Could you check a few things on this model? Use its own coordinates, in mm. A direction names the side the tool comes from. Give positions to 0.01 mm unless a question says otherwise; leave off trailing zeros. Write each loop counter-clockwise with the first axis right and the second up, starting at its lowest first coordinate (ties: lowest second). Pieces come first, ordered by that corner, then holes. Notation, with made-up numbers: (71.25, 7.25) - (85.25, 7.25) arc R32 ccw to (85.25, 33.25) - close; hole circle Ø8 at (-12, -14.75). An arc over 180 degrees is marked (long way). Answer in a Markdown table with one row per item.
from build123d import *
from OCP.BRepFilletAPI import BRepFilletAPI_MakeChamfer

# Parameters (mm, degrees)
ESTRUSIONE_ESTRUSIONE1_DEPTH                         = 66
RACCORDO1_R                                          = 10
SMUSSO1_SIZE                                         = 2
SMUSSO1_SIZE2                                        = 2.155800013
SMUSSO1_SIZE2_2                                      = 1.873732722
SMUSSO2_SIZE                                         = 5
FORO_LAMATO_PER_VITE_M4_A_TESTA_CILINDRI_D           = 4.5
FORO_LAMATO_PER_VITE_M4_A_TESTA_CILINDRI_DEPTH       = 30
FORO_LAMATO_PER_VITE_M4_A_TESTA_CILINDRI_CBORE_D     = 10
FORO_LAMATO_PER_VITE_M4_A_TESTA_CILINDRI_CBORE_DEPTH = 3
FORO_LAMATO_PER_VITE_M4_A_TESTA_CILINDRI_TIP         = 1.351936393
FORO_LAMATO_PER_VITE_M4_A_TESTA_CILI_2_D             = 4.5
FORO_LAMATO_PER_VITE_M4_A_TESTA_CILI_2_DEPTH         = 30
FORO_LAMATO_PER_VITE_M4_A_TESTA_CILI_2_CBORE_D       = 10
FORO_LAMATO_PER_VITE_M4_A_TESTA_CILI_2_CBORE_DEPTH   = 10
FORO_LAMATO_PER_VITE_M4_A_TESTA_CILI_2_TIP           = 1.351936393
FORO_LAMATO_PER_VITE_M4_A_TESTA_CILI_3_D             = 4.5
FORO_LAMATO_PER_VITE_M4_A_TESTA_CILI_3_DEPTH         = 45
FORO_LAMATO_PER_VITE_M4_A_TESTA_CILI_3_CBORE_D       = 10
FORO_LAMATO_PER_VITE_M4_A_TESTA_CILI_3_CBORE_DEPTH   = 32
FORO_LAMATO_PER_VITE_M4_A_TESTA_CILI_3_TIP           = 1.351936393


with BuildPart() as part:
    # Schizzo1 → Estrusione-Estrusione1 (new body)
    with BuildSketch(Plane.XY):
        Polygon((25.25, 100), (32.25, 100), (39.25, 0), (-39.25, 0), (-64.110342, 0), (-64.110342, 114.69), (-25.25, 114.69), (-25.25, 100), (-25.25, 15), (25.25, 15), align=None)
    extrude(amount=ESTRUSIONE_ESTRUSIONE1_DEPTH)

    # Raccordo1
    raccordo1_edges = [part.edges().sort_by_distance(p)[0] for p in [
        (-25.25, 15, 33),
        (25.25, 15, 33),
    ]]
    fillet(raccordo1_edges, radius=RACCORDO1_R)

    # Smusso1: one chamfer whose edges measure the first distance from different faces: ONE call of the kernel's chamfer builder (chamfer() names one face for all edges)
    smusso1_edges_1 = [part.edges().sort_by_distance(p)[0] for p in [
        (35.75, 50, 0),
        (-12.430171, 0, 0),
        (-64.110342, 57.345, 0),
        (-44.680171, 114.69, 0),
        (25.25, 62.5, 0),
        (25.25, 100, 33),
        (-44.680171, 114.69, 66),
        (-64.110342, 57.345, 66),
        (-12.430171, 0, 66),
        (-25.25, 69.845, 0),
        (-25.25, 69.845, 66),
        (0, 15, 0),
        (0, 15, 66),
        (-22.321067812, 17.928932188, 0),
        (-22.321067812, 17.928932188, 66),
        (35.75, 50, 66),
        (22.321067812, 17.928932188, 0),
        (22.321067812, 17.928932188, 66),
        (25.25, 62.5, 66),
    ]]
    smusso1_edges_2 = [part.edges().sort_by_distance(p)[0] for p in [
        (32.25, 100, 33),
    ]]
    smusso1_side_2 = [part.faces().sort_by_distance(p)[0] for p in [
        (35.75, 50, 33),
    ]]
    smusso1_edges_3 = [part.edges().sort_by_distance(p)[0] for p in [
        (39.25, 0, 33),
    ]]
    smusso1_side_3 = [part.faces().sort_by_distance(p)[0] for p in [
        (-12.430171, 0, 33),
    ]]
    smusso1 = BRepFilletAPI_MakeChamfer(part.part.solid().wrapped)
    for e in smusso1_edges_1:
        smusso1.Add(SMUSSO1_SIZE, e.wrapped)
    for e in smusso1_edges_2:
        smusso1.Add(SMUSSO1_SIZE, SMUSSO1_SIZE2, e.wrapped, smusso1_side_2[0].wrapped)  # the first distance lies on this face
    for e in smusso1_edges_3:
        smusso1.Add(SMUSSO1_SIZE, SMUSSO1_SIZE2_2, e.wrapped, smusso1_side_3[0].wrapped)  # the first distance lies on this face
    add(Compound.cast(smusso1.Shape()), mode=Mode.REPLACE)

    # Smusso2
    # the kernel refuses this chamfer: 5 mm, written as the material it takes off along each edge
    with BuildSketch(Plane(origin=(14.39158506, 100, 66), x_dir=(2.02935454733688e-15, -0.9996219169112968, 0.027495876610587663), z_dir=(1, 0, 0)), Plane(origin=(14.39158506, 100, 0), x_dir=(0, 0.0274958766105877, 0.9996219169112968), z_dir=(1, 0, 0))) as smusso2_piece_1:
        Polygon((SMUSSO2_SIZE * 0.999621916911, SMUSSO2_SIZE * 0.0274958766106), (-SMUSSO2_SIZE * 0.0274958766106, SMUSSO2_SIZE * 0.999621916911), (0, 0), align=None)
    extrude(amount=28.561029867, mode=Mode.SUBTRACT)

    # Foro lamato per Vite M4 a testa cilindri
    with Locations(Plane(origin=(35.25, 0, 0), x_dir=(0, 0, 1), z_dir=(1, 0, 0))):
        with Locations((56, -85.613628), (10, -85.613628)):
            CounterBoreHole(FORO_LAMATO_PER_VITE_M4_A_TESTA_CILINDRI_D / 2, FORO_LAMATO_PER_VITE_M4_A_TESTA_CILINDRI_CBORE_D / 2, FORO_LAMATO_PER_VITE_M4_A_TESTA_CILINDRI_CBORE_DEPTH, depth=FORO_LAMATO_PER_VITE_M4_A_TESTA_CILINDRI_DEPTH)
            with Locations((0, 0, -(FORO_LAMATO_PER_VITE_M4_A_TESTA_CILINDRI_DEPTH + FORO_LAMATO_PER_VITE_M4_A_TESTA_CILINDRI_TIP / 2))):  # 118° drill point
                Cone(0, FORO_LAMATO_PER_VITE_M4_A_TESTA_CILINDRI_D / 2, FORO_LAMATO_PER_VITE_M4_A_TESTA_CILINDRI_TIP, mode=Mode.SUBTRACT)

    # Foro lamato per Vite M4 a testa cili 2
    with Locations(Plane(origin=(0, 15, 0), x_dir=(1, 0, 0), z_dir=(0, 1, 0))):
        with Locations((-10.245584981, -33), (9.754415019, -33)):
            CounterBoreHole(FORO_LAMATO_PER_VITE_M4_A_TESTA_CILI_2_D / 2, FORO_LAMATO_PER_VITE_M4_A_TESTA_CILI_2_CBORE_D / 2, FORO_LAMATO_PER_VITE_M4_A_TESTA_CILI_2_CBORE_DEPTH, depth=FORO_LAMATO_PER_VITE_M4_A_TESTA_CILI_2_DEPTH)
            with Locations((0, 0, -(FORO_LAMATO_PER_VITE_M4_A_TESTA_CILI_2_DEPTH + FORO_LAMATO_PER_VITE_M4_A_TESTA_CILI_2_TIP / 2))):  # 118° drill point
                Cone(0, FORO_LAMATO_PER_VITE_M4_A_TESTA_CILI_2_D / 2, FORO_LAMATO_PER_VITE_M4_A_TESTA_CILI_2_TIP, mode=Mode.SUBTRACT)

    # Foro lamato per Vite M4 a testa cili 3
    with Locations(Plane.ZY.offset(64.110342)):
        with Locations((10, 85.613628), (56, 85.613628)):
            CounterBoreHole(FORO_LAMATO_PER_VITE_M4_A_TESTA_CILI_3_D / 2, FORO_LAMATO_PER_VITE_M4_A_TESTA_CILI_3_CBORE_D / 2, FORO_LAMATO_PER_VITE_M4_A_TESTA_CILI_3_CBORE_DEPTH, depth=FORO_LAMATO_PER_VITE_M4_A_TESTA_CILI_3_DEPTH)
            with Locations((0, 0, -(FORO_LAMATO_PER_VITE_M4_A_TESTA_CILI_3_DEPTH + FORO_LAMATO_PER_VITE_M4_A_TESTA_CILI_3_TIP / 2))):  # 118° drill point
                Cone(0, FORO_LAMATO_PER_VITE_M4_A_TESTA_CILI_3_D / 2, FORO_LAMATO_PER_VITE_M4_A_TESTA_CILI_3_TIP, mode=Mode.SUBTRACT)


solid = part.part
1) Imagine slicing it at C-C (y = 9). List the corners of the cut face in (x, z) for me, then the cut area to 3 significant figures.
Check values:
| item | result |
|---|---|
| outline | (-64.11, 2) - (-62.11, 0) - (36.62, 0) - (38.62, 2) - (38.62, 64) - (36.62, 66) - (-62.11, 66) - (-64.11, 64) - close; hole circle Ø10 at (-10.25, 33); hole circle Ø10 at (9.75, 33) |
| area | 6,620 mm2 |
2) On a 3-axis mill with a long thin cutter (end or side, diameter ignored), from which of +Z, -Z, +X, -X, +Y, -Y can I reach the whole of each face in a straight line? I mean faces 5 (the face through (32.815, 80.656, 55.349)), 6 (the face through (29, 98, 3)), 7 (the face through (-22.786, 17.628, 1.458)). Say none if no direction works.
Check values:
| item | result |
|---|---|
| face 5 | +X |
| face 6 | -Z, +X, +Y |
| face 7 | -Z, +Y |
3) Imagine slicing it at A-A (z = 33). State how many separate pieces and enclosed holes the cut face has, then the cut area to 3 significant figures.
Check values:
| item | result |
|---|---|
| separate pieces | 3 |
| enclosed holes | 0 |
| area | 6,060 mm2 |
4) Will these pins go through, and if not, where does the flat tip stop? P1, Ø11.5, axis at x = -10.25, z = 33, coming from the +Y side; P2, Ø8, axis at y = 86, z = 54.5, coming from the +X side; P3, Ø5, axis at y = 41.5, z = 49, coming from the +X side.
Check values:
| item | result |
|---|---|
| P1 | stops at y = 15.03 |
| P2 | stops at x = 33.42 |
| P3 | stops at x = 36.52 |
5) Imagine slicing it at D-D (x = -38.5). List the corners of the cut face in (y, z) for me, then the cut area to 3 significant figures.
Check values:
| item | result |
|---|---|
| outline | (0, 2) - (2, 0) - (112.69, 0) - (114.69, 2) - (114.69, 64) - (112.69, 66) - (2, 66) - (0, 64) - close; hole circle Ø10 at (85.61, 10); hole circle Ø10 at (85.61, 56) |
| area | 7,400 mm2 |
6) If I drill on line 1 (Y direction, x = -46, z = 56); line 2 (X direction, y = 88, z = 7); line 3 (Y direction, x = 30, z = 56), over which ranges is the centre line in solid material (lowest first)?
Check values:
| item | result |
|---|---|
| line 1 | y = 0 to 80.61, 90.61 to 114.69 |
| line 2 | x = -32.11 to -25.25, 25.25 to 32.25 |
| line 3 | y = 0 to 83.36, 87.86 to 100 |
7) Imagine slicing it at B-B (z = 21.5). List the corners of the cut face in (x, y) for me, then the cut area to 3 significant figures.
Check values:
| item | result |
|---|---|
| outline | (-64.11, 0) - (37.25, 0) - (39.12, 1.87) - (32.39, 98) - (30.09, 100) - (27.25, 100) - (25.25, 98) - (25.25, 25) arc R10 cw to (15.25, 15) - (-15.25, 15) arc R10 cw to (-25.25, 25) - (-25.25, 114.69) - (-64.11, 114.69) - close |
| area | 6,300 mm2 |
8) We'd pull the mould along Y, two halves only. Please class faces 1 (the face through (-48.334, 87.115, 14.769)), 2 (the face through (25.25, 61, 33)), 3 (the face through (28.7, 87.81, 10.49)), 4 (the face through (-45, 114.69, 33)): +Y half, -Y half, draft (parallel to the pull), parting line (faces both ways), or undercut.
Check values:
| item | result |
|---|---|
| face 1 | undercut |
| face 2 | draft |
| face 3 | undercut |
| face 4 | +Y half |
